Here's the drawing with two shaded views (mm, measured from the low corner). I have some questions. A direction names the side the tool comes from. Give positions to 0.01 mm unless a question says otherwise; leave off trailing zeros. Order: outer loops, then holes, each group sorted by start corner. A loop starts at its lowest first (then second) coordinate and runs counter-clockwise, first axis right, second up. Notation, with made-up numbers: M -17,88.5 L -11,88.5 A25 cw -11,112.5 Z; hole C 16,57 d1. An arc over 180 degrees is marked long. One line per question, with ' | ' between items. Start each with the question number.
1) Thinking about a two-plate mould opening in X: for the marked faces 1, 2 and 3, which applies, +X half, -X half, draft (parallel to the pull), parting line (faces both ways), or undercut?
2) For the marked faces 4 and 5, which set-ups out of +Z, -Z, +X, -X, +Y, -Y let a thin tool reach every point of the face, with its end or its side?
3) If we section it at D-D, the plane z = 32.5: Please give me the cut outline in (x, y), plus the area to 3 significant figures.
4) If we section it at C-C, the plane x = 12.5: Please give me the cut outline in (y, z), plus the area to 3 significant figures.
5) If we section it at A-A, the plane y = 62.5: Please give me the cut outline in (x, z).
6) I'm going to push a flat-ended pin straight in: pin 1 Ø3.5 at (x, y) = (10, 112.5) entering from -Z. Where does the tip first touch, or does it pass through?
7) If we section it at B-B, the plane z = 8: Please give me the cut outline in (x, y), plus the area to 3 significant figures.
8) Please list where these lines run through material, in increasing order: line 1 along Y through (x, z) = (12.5, 4.5); line 2 along X through (y, z) = (62.5, 29.5); line 3 along X through (y, z) = (62.5, 4.5). Write a range as [from, to].
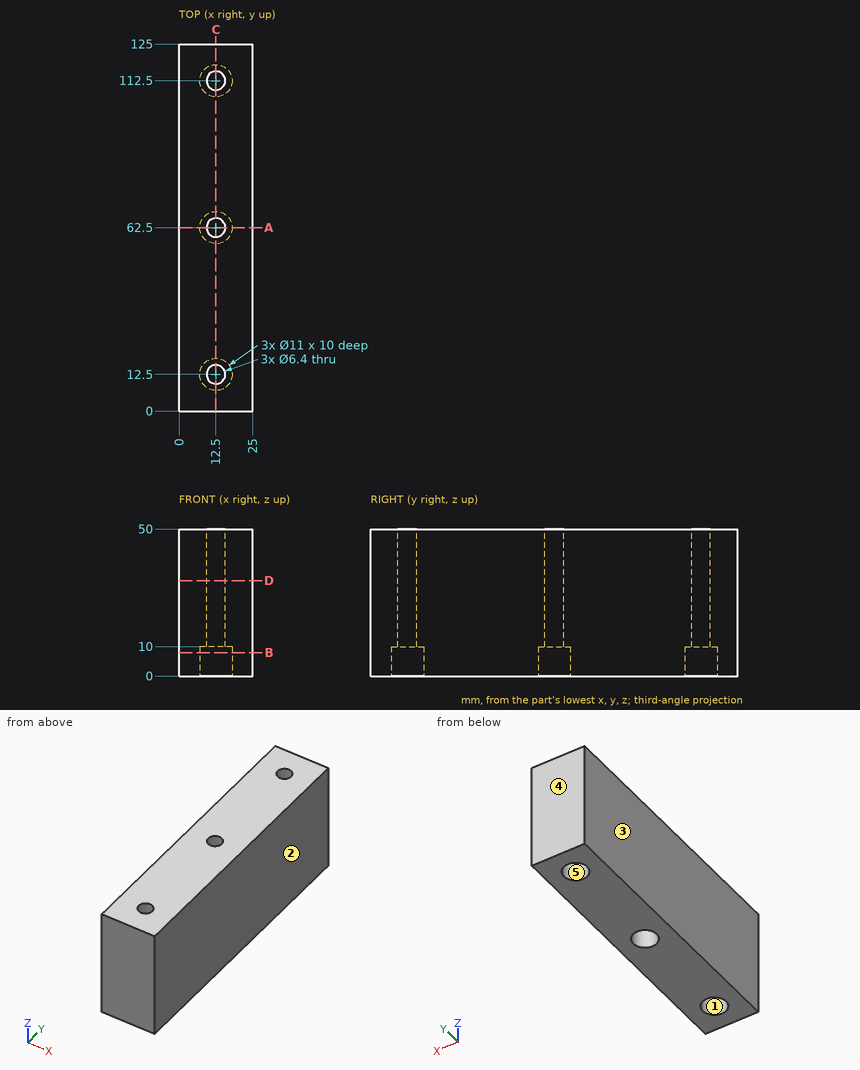
Results found:
1) face 1: undercut | face 2: +X half | face 3: -X half
2) face 4: +Z, -Z, +X, -X, +Y | face 5: -Z
3) outline: M 0,0 L 25,0 L 25,125 L 0,125 Z; hole C 12.5,12.5 d6.4; hole C 12.5,62.5 d6.4; hole C 12.5,112.5 d6.4 | area: 3,030 mm²
4) outline: M 0,0 L 7,0 L 7,10 L 9.3,10 L 9.3,50 L 0,50 Z; M 15.7,10 L 18,10 L 18,0 L 57,0 L 57,10 L 59.3,10 L 59.3,50 L 15.7,50 Z; M 65.7,10 L 68,10 L 68,0 L 107,0 L 107,10 L 109.3,10 L 109.3,50 L 65.7,50 Z; M 115.7,10 L 118,10 L 118,0 L 125,0 L 125,50 L 115.7,50 Z | area: 5,150 mm²
5) outline: M 0,0 L 7,0 L 7,10 L 9.3,10 L 9.3,50 L 0,50 Z; M 15.7,10 L 18,10 L 18,0 L 25,0 L 25,50 L 15.7,50 Z
6) pin 1: stops at z = 10
7) outline: M 0,0 L 25,0 L 25,125 L 0,125 Z; hole C 12.5,12.5 d11; hole C 12.5,62.5 d11; hole C 12.5,112.5 d11 | area: 2,840 mm²
8) line 1: y = [0, 7], [18, 57], [68, 107], [118, 125] | line 2: x = [0, 9.3], [15.7, 25] | line 3: x = [0, 7], [18, 25]
